For this review, take the finished solid that the model builds, in its own axes (mm). A direction names the side the tool comes from. Coordinates: 2 decimals unless noted, no trailing zeros. Write each loop counter-clockwise with the first axis right and the second up, starting at its lowest first coordinate (ties: lowest second). Pieces come first, ordered by that corner, then holes. Notation, with made-up numbers: M 87,-36.75 L 107,-36.75 A9 cw 107,-27.75 Z; hole C 5,80 d6. An arc over 180 degrees is marked long. One line per question, with ' | ' between items.
from build123d import *

# Parameters (mm, degrees)
TAGLIO_ESTRUSIONE1_REACH      = 19.096
TAGLIO_ESTRUSIONE1_END_RADIUS = 10.5
SCHIZZO2_R                    = 1.5
TAGLIO_ESTRUSIONE2_REACH      = 19.096
TAGLIO_ESTRUSIONE2_END_RADIUS = 10.5
SCHIZZO3_R                    = 1.5


with BuildPart() as part:
    # Schizzo1 → Rivoluzione1 (revolve)
    with BuildSketch(Plane.XY, mode=Mode.PRIVATE) as rivoluzione1_sk:
        Polygon((-8, 3), (-7.5, 2.5), (7.5, 2.5), (8, 3), (8, 10), (7.5, 10.5), (0.524062064, 10.5), (0.01763809, 8.61), (-7.48236191, 8.61), (-7.988785883, 10.5), (-8.471748797, 10.370590477), (-8, 8.61), align=None)
    revolve(rivoluzione1_sk.sketch.rotate(Axis((-8, 0, 0), (1, 0, 0)), 180), axis=Axis((-8, 0, 0), (1, 0, 0)))

    # Taglio-Estrusione1: up to this cylinder (the profile starts inside it)
    taglio_estrusione1_end = Plane(origin=(3.75, 0, 0), z_dir=(-1, 0, 0)) * Cylinder(TAGLIO_ESTRUSIONE1_END_RADIUS, 60.192, mode=Mode.PRIVATE)
    # Schizzo2 → Taglio-Estrusione1 (cut, up to the surface)
    with BuildSketch(Plane.XY, mode=Mode.PRIVATE) as taglio_estrusione1_sk1:
        with Locations((3.75, 0)):
            Circle(SCHIZZO2_R)
    taglio_estrusione1_tool1 = extrude(taglio_estrusione1_sk1.sketch, amount=-TAGLIO_ESTRUSIONE1_REACH, mode=Mode.PRIVATE) & taglio_estrusione1_end
    add(taglio_estrusione1_tool1.solids().sort_by_distance((3.75, 0, 0))[0], mode=Mode.SUBTRACT)

    # Taglio-Estrusione2: up to this cylinder (the profile starts inside it)
    taglio_estrusione2_end = Plane(origin=(4.012031, 0, 0), z_dir=(-1, 0, 0)) * Cylinder(TAGLIO_ESTRUSIONE2_END_RADIUS, 60.192, mode=Mode.PRIVATE)
    # Schizzo3 → Taglio-Estrusione2 (cut, up to the surface)
    with BuildSketch(Plane(origin=(0, 0, 0), x_dir=(1, 0, 0), z_dir=(0, 1, 0)), mode=Mode.PRIVATE) as taglio_estrusione2_sk1:
        with Locations(Location((4.012031032, 0, 0), (0, 0, 270))):
            Circle(SCHIZZO3_R)
    taglio_estrusione2_tool1 = extrude(taglio_estrusione2_sk1.sketch, amount=-TAGLIO_ESTRUSIONE2_REACH, mode=Mode.PRIVATE) & taglio_estrusione2_end
    add(taglio_estrusione2_tool1.solids().sort_by_distance((4.012031, 0, 0))[0], mode=Mode.SUBTRACT)


solid = part.part
1) Machinability: for faces 1 (the flat face through (-8, -4, 0)), 2 (the cylindrical face through (3.963, -4.845, 9.315)), 3 (the cylindrical face through (3.438, -6.191, 1.386)), which of the approach directions +Z, -Z, +X, -X, +Y, -Y give a long, thin tool a straight path to every point of the face, cutting with its end or side? Answer none if there is none.
Responses:
face 1: -X | face 2: +X, -X | face 3: -Y
2) The part is to be moulded in two halves that separate along Z. For faces 4 (the cylindrical face through (-3.785, 1.866, 8.405)), 5 (the cylindrical face through (2.25, 0.07, -6.19)), 6 (the cylindrical face through (0.1, 2, 1.5)), say which applies: +Z half, -Z half, draft (parallel to the pull), parting line (faces both ways), or undercut.
Responses:
face 4: parting line | face 5: draft | face 6: undercut
3) Insertion check: pin 1 Ø2 at (x, z) = (-6, 1.5) entering from -Y; pin 2 Ø1 at (x, y) = (2.5, -1) entering from +Z; pin 3 Ø6 at (x, z) = (-1.5, 6.5) entering from +Y; pin 4 Ø8 at (x, z) = (3.5, -0.5) entering from +Y. Each pin has a flat end and moves straight along its axis. Give the tip position at first contact, or say it passes through.
Responses:
pin 1: y = -8.6 | pin 2: z = 10.49 | pin 3: y = 9.59 | pin 4: y = 10.5
4) To check wall thickness, follow line 1 along X through (y, z) = (0, -8); line 2 along X through (y, z) = (3.75, 3.25); line 3 along Z through (x, y) = (3, 0). State the ranges of each line that lie inside material, in increasing order. Write a range as [from, to].
Responses:
line 1: [-8, 2.25], [5.25, 8] | line 2: [-8, 8] | line 3: [2.5, 10.5]
5) We need section C-C on x = -4.5. State the section outline as (y, z) points.
Responses:
outline: C 0,0 d17.22; hole C 0,0 d5
6) We need section B-B on z = 0. State the section outline as (x, y) points, then the cut area to 3 significant figures.
Responses:
outline: M -8.47,-10.37 L -7.99,-10.5 L -7.48,-8.61 L 0.02,-8.61 L 0.52,-10.5 L 2.51,-10.5 L 2.51,-2.5 L -7.5,-2.5 L -8,-3 L -8,-8.61 Z; M -8.47,10.37 L -8,8.61 L -8,3 L -7.5,2.5 L 7.5,2.5 L 8,3 L 8,10 L 7.5,10.5 L 0.52,10.5 L 0.02,8.61 L -7.48,8.61 L -7.99,10.5 Z; M 5.51,-10.5 L 7.5,-10.5 L 8,-10 L 8,-3 L 7.5,-2.5 L 5.51,-2.5 Z | area: 202 mm^2
7) We need section A-A on y = 0. State the section outline as (x, z) points.
Responses:
outline: M -8.47,-10.37 L -7.99,-10.5 L -7.48,-8.61 L 0.02,-8.61 L 0.52,-10.5 L 2.25,-10.5 L 2.25,-2.5 L -7.5,-2.5 L -8,-3 L -8,-8.61 Z; M -8.47,10.37 L -8,8.61 L -8,3 L -7.5,2.5 L 7.5,2.5 L 8,3 L 8,10 L 7.5,10.5 L 0.52,10.5 L 0.02,8.61 L -7.48,8.61 L -7.99,10.5 Z; M 5.25,-10.5 L 7.5,-10.5 L 8,-10 L 8,-3 L 7.5,-2.5 L 5.25,-2.5 Z
